Autodesk Inventor part; units mm, degrees
ref_plane "YZ Plane" through (0, 0, 0) normal (1, 0, 0) x (0, 1, 0)
ref_plane "XZ Plane" through (0, 0, 0) normal (0, 1, 0) x (-1, 0, 0)
ref_plane "XY Plane" through (0, 0, 0) normal (0, 0, 1) x (1, 0, 0)
sketch "Sketch1" plane through (0, 0, 0) normal (0, 1, 0) x (-1, 0, 0)
  circle A0 centre (0, 0) radius 19
  circle A1 centre (0, 0) radius 10.5
  dimension "d0" = 38
  dimension "d1" = 21
extrude "Extrusion1" add sketch "Sketch1" along normal blind 5
sketch "Sketch2" plane through (0, 5, 0) normal (0, 1, 0) x (1, 0, 0)
  circle A0 centre (0, 0) radius 14 construction
  point P0 (-14, 0)
  dimension "d4" = 28
hole "Hole1" at (-14, 5, 0) direction (0, -1, 0) diameter 2.459 depth 5
pattern_circular "Circular Pattern1" count 8 over 360 about axis through (0, 0, 0) along (0, 1, 0) of "Hole1"
properties part number "212"
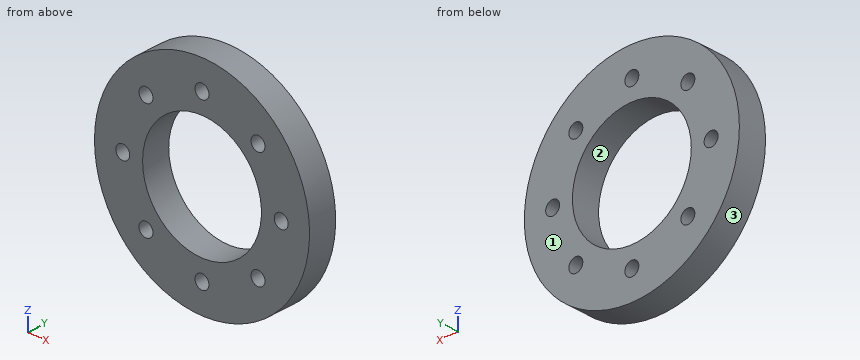
Input: part model. Units: mm. Frame: model coordinates. Face numbers are marked on the shaded views. Coordinates: 2 decimals unless noted, no trailing zeros. Write each loop counter-clockwise with the first axis right and the second up, starting at its lowest first coordinate (ties: lowest second). Pieces come first, ordered by that corner, then holes. Notation, with made-up numbers: M 59,88 L 65,88 A25 ccw 65,107 Z; hole C 59,71.25 d8. An arc over 180 degrees is marked long. Answer as a JSON object with one key per item and string values. Group by question number.
(1) Contact query for flat-ended pins moving along their axis: P1, Ø2, axis at x = 9.9, z = 9.9, coming from the -Y side; P2, Ø3, axis at y = 2, z = -4, coming from the -X side. Output: stop coordinate, or through.
(2) Mould query, pull axis Z, two halves, no side actions, for the marked faces 1, 2 and 3. Classes: pulls with the +Z half, pulls with the -Z half, needs draft (parallel to the pull), parting line crosses it, or undercut.
(3) Section C-C on y = 1.9. Give the number of separate pieces and of enclosed holes in the cut face, plus the area to 3 significant figures.
(4) Section B-B on z = 4.5. Output: boundary loops of the cut face in (x, y), plus the area to 3 significant figures.
(5) Ray query, line 1 along Z through (x, y) = (0, 1.3); line 2 along X through (y, z) = (3.85, -9.5); line 3 along X through (y, z) = (1.15, -8.5). Return the intervals inside material, ascending. Write a range as [from, to].
(6) Section A-A on x = -6. Output: boundary loops of the cut face in (y, z), plus the area to 3 significant figures.
Result set:
{
 "1": {"P1": "passes through", "P2": "stops at x = -18.83"},
 "2": {"face 1": "needs draft", "face 2": "undercut", "face 3": "parting line crosses it"},
 "3": {"separate pieces": "1", "enclosed holes": "9", "area": "750 mm2"},
 "4": {"outline": "M -18.46,0 L -9.49,0 L -9.49,5 L -18.46,5 Z; M 9.49,0 L 18.46,0 L 18.46,5 L 9.49,5 Z", "area": "89.7 mm2"},
 "5": {"line 1": "z = [-19, -15.23], [-12.77, -10.5], [10.5, 12.77], [15.23, 19]", "line 2": "x = [-16.45, -11.06], [-8.74, -4.47], [4.47, 8.74], [11.06, 16.45]", "line 3": "x = [-16.99, -6.16], [6.16, 16.99]"},
 "6": {"outline": "M 0,-18.03 L 5,-18.03 L 5,-8.62 L 0,-8.62 Z; M 0,8.62 L 5,8.62 L 5,18.03 L 0,18.03 Z", "area": "94.1 mm2"}
}
